from build123d import *

# Parameters (mm, degrees)
SKETCH1_W           = 150
SKETCH1_H           = 84
SKETCH1_R           = 12
SKETCH1_R_2         = 6.25
SKETCH1_R_3         = 1.5
BOSS_EXTRUDE2_DEPTH = 3


with BuildPart() as part:
    # Sketch1 → Boss-Extrude2 (new body)
    with BuildSketch(Plane(origin=(0, 0, 0), x_dir=(1, 0, 0), z_dir=(0, 1, 0))):
        with Locations((14.43134335, 3.286639095)):
            Rectangle(SKETCH1_W, SKETCH1_H)
        with Locations(Location((-41.06865665, -17.963360905, 0), (0, 0, 270))):
            Circle(SKETCH1_R, mode=Mode.SUBTRACT)
        with Locations(Location((-4.06865665, -17.963360905, 0), (0, 0, 270))):
            Circle(SKETCH1_R, mode=Mode.SUBTRACT)
        with Locations(Location((-34.31865665, 15.286639095, 0), (0, 0, 270))):
            Circle(SKETCH1_R_2, mode=Mode.SUBTRACT)
        with Locations(Location((-21.56865665, 15.286639095, 0), (0, 0, 270))):
            Circle(SKETCH1_R_3, mode=Mode.SUBTRACT)
        with Locations(Location((-2.81865665, 15.286639095, 0), (0, 0, 270))):
            Circle(SKETCH1_R_2, mode=Mode.SUBTRACT)
        with Locations(Location((9.43134335, 18.786639095, 0), (0, 0, 270))):
            Circle(SKETCH1_R_3, mode=Mode.SUBTRACT)
        with Locations(Location((9.43134335, 11.786639095, 0), (0, 0, 270))):
            Circle(SKETCH1_R_3, mode=Mode.SUBTRACT)
        with Locations(Location((69.93134335, -17.963360905, 0), (0, 0, 90))):
            Circle(SKETCH1_R, mode=Mode.SUBTRACT)
        with Locations(Location((32.93134335, -17.963360905, 0), (0, 0, 90))):
            Circle(SKETCH1_R, mode=Mode.SUBTRACT)
        with Locations(Location((19.43134335, 11.786639095, 0), (0, 0, 90))):
            Circle(SKETCH1_R_3, mode=Mode.SUBTRACT)
        with Locations(Location((19.43134335, 18.786639095, 0), (0, 0, 90))):
            Circle(SKETCH1_R_3, mode=Mode.SUBTRACT)
        with Locations(Location((31.68134335, 15.286639095, 0), (0, 0, 90))):
            Circle(SKETCH1_R_2, mode=Mode.SUBTRACT)
        with Locations(Location((50.43134335, 15.286639095, 0), (0, 0, 90))):
            Circle(SKETCH1_R_3, mode=Mode.SUBTRACT)
        with Locations(Location((63.18134335, 15.286639095, 0), (0, 0, 90))):
            Circle(SKETCH1_R_2, mode=Mode.SUBTRACT)
    extrude(amount=-BOSS_EXTRUDE2_DEPTH)


solid = part.part
Could you check a few things on this model? Use its own coordinates, in mm. Give positions to 0.01 mm unless a question says otherwise; leave off trailing zeros. Order: outer loops, then holes, each group sorted by start corner. A loop starts at its lowest first (then second) coordinate and runs counter-clockwise, first axis right, second up. Notation, with made-up numbers: (64, -34) -> (91, -34) arc R27 cw to (91, 5) -> close; hole circle Ø2 at (24, -8.75). An arc over 180 degrees is marked (long way). Return JSON: item names as keys, results as strings.
1. Imagine slicing it at A-A on x = 67. List the corners of the cut face in (y, z) for me, then the cut area to 3 significant figures.
Answer list:
{"outline": "(-3, -45.29) -> (0, -45.29) -> (0, -20.23) -> (-3, -20.23) -> close; (-3, -10.34) -> (0, -10.34) -> (0, 6.33) -> (-3, 6.33) -> close; (-3, 29.6) -> (0, 29.6) -> (0, 38.71) -> (-3, 38.71) -> close", "area": "152 mm2"}
2. I need wall thicknesses on line 1 (Z direction, x = 9.5, y = -1.35); line 2 (X direction, y = -1.3, z = 15.5); line 3 (Z direction, x = 29.5, y = -2.45). Which ranges of each line are inside material? Lowest first, please. Write a range as from..to.
Answer list:
{"line 1": "z = -45.29..-20.29, -17.29..-13.29, -10.29..38.71", "line 2": "x = -60.57..-52.81, -29.32..-15.81, 7.68..21.19, 44.68..58.19, 81.68..89.43", "line 3": "z = -45.29..-21.14, -9.43..6.46, 29.46..38.71"}
3. Thinking about a two-plate mould opening in Z: for faces 1 (the cylindrical face through (-21.118, -1.479, -13.856)), 2 (the flat face through (-60.569, -1, -3)), 3 (the cylindrical face through (10.92, -1.48, -18.98)), 4 (the flat face through (13, -1, 38.713)), which applies, pulls with the +Z half, pulls with the -Z half, needs draft (parallel to the pull), parting line crosses it, or undercut?
Answer list:
{"face 1": "undercut", "face 2": "needs draft", "face 3": "undercut", "face 4": "pulls with the +Z half"}
4. Imagine slicing it at C-C on y = -0.65. Give the number of separate pieces and of enclosed holes in the cut face, then the cut area to 3 significant figures.
Answer list:
{"separate pieces": "1", "enclosed holes": "14", "area": "10,300 mm2"}
5. Imagine slicing it at D-D on z = 27. List the corners of the cut face in (x, y) for me.
Answer list:
{"outline": "(-60.57, -3) -> (-48.96, -3) -> (-48.96, 0) -> (-60.57, 0) -> close; (-33.17, -3) -> (-11.96, -3) -> (-11.96, 0) -> (-33.17, 0) -> close; (3.83, -3) -> (25.04, -3) -> (25.04, 0) -> (3.83, 0) -> close; (40.83, -3) -> (62.04, -3) -> (62.04, 0) -> (40.83, 0) -> close; (77.83, -3) -> (89.43, -3) -> (89.43, 0) -> (77.83, 0) -> close"}
6. Imagine slicing it at B-B on x = -48.5. List the corners of the cut face in (y, z) for me.
Answer list:
{"outline": "(-3, -45.29) -> (0, -45.29) -> (0, 8.54) -> (-3, 8.54) -> close; (-3, 27.39) -> (0, 27.39) -> (0, 38.71) -> (-3, 38.71) -> close"}
